Answer from the drawing. Dimensions are ordinates in mm from the lowest x, y and z of the part. Round coordinates to 2 decimals unless told otherwise and drop trailing zeros. Order: outer loops, then holes, each group sorted by start corner. A loop starts at its lowest first (then second) coordinate and runs counter-clockwise, first axis right, second up.
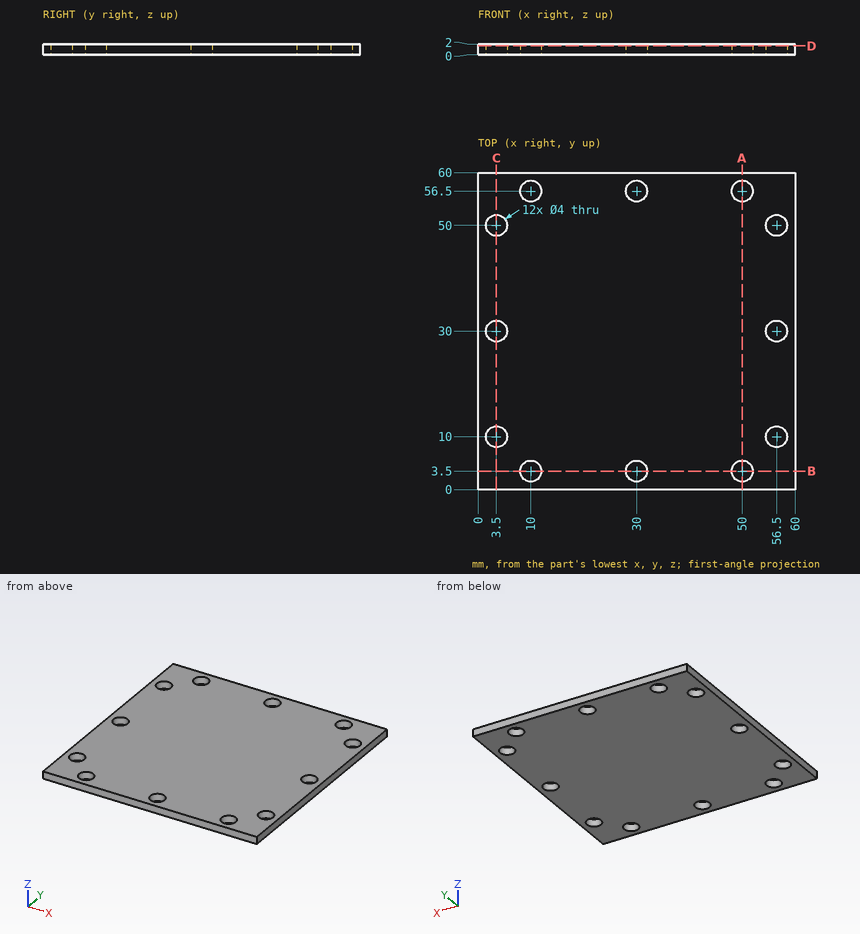
Q1. A cutting plane is placed at A-A, the plane x = 50. Give the vertices of the cut face in (y, z).
Outcome:
outline: (0, 0) - (1.5, 0) - (1.5, 2) - (0, 2) - close; (5.5, 0) - (54.5, 0) - (54.5, 2) - (5.5, 2) - close; (58.5, 0) - (60, 0) - (60, 2) - (58.5, 2) - close
Q2. Straight lines are drawn through the part: probe 1 along Y at (x, z) = (50, 1.15); probe 2 along X at (y, z) = (3.5, 1.6). For each, find the intervals that lie inside material, in ascending order.
Outcome:
probe 1: y = 0 to 1.5, 5.5 to 54.5, 58.5 to 60
probe 2: x = 0 to 8, 12 to 28, 32 to 48, 52 to 60
Q3. A cutting plane is placed at B-B, the plane y = 3.5. Give the vertices of the cut face in (x, z).
Outcome:
outline: (0, 0) - (8, 0) - (8, 2) - (0, 2) - close; (12, 0) - (28, 0) - (28, 2) - (12, 2) - close; (32, 0) - (48, 0) - (48, 2) - (32, 2) - close; (52, 0) - (60, 0) - (60, 2) - (52, 2) - close
Q4. A flat-ended cylindrical pin translates along its axis: pin 1 (6.5 mm diameter, centred on x = 3.5, y = 50, fed in from +Z). Find the tip coordinate at first contact, or state that the pin passes through.
Outcome:
pin 1: stops at z = 2
Q5. A cutting plane is placed at D-D, the plane z = 1.65. Give the number of separate pieces and of enclosed holes in the cut face, plus the area to 3 significant figures.
Outcome:
separate pieces: 1
enclosed holes: 12
area: 3,450 mm2
